```python
from build123d import *

# Parameters (mm, degrees)
F0_R          = 30
F0_R_2        = 3.625
F0_R_3        = 11.1
F2_DEPTH      = 3.25
F2_DEPTH_BACK = 3.25
F1_R          = 40
F1_R_2        = 30
F3_DEPTH      = 5
F3_DEPTH_BACK = 5


with BuildPart() as f2:
    # F0 (on Top) → F2 (new body, two sides)
    with BuildSketch(Plane.XY) as f2_sk:
        Circle(F0_R)
        with Locations((-6.983624, -20.439105)):
            Circle(F0_R_2, mode=Mode.SUBTRACT)
        with Locations((-20.439105, -6.983624)):
            Circle(F0_R_2, mode=Mode.SUBTRACT)
        with Locations((-11.348298, -11.348298)):
            Circle(F0_R_2, mode=Mode.SUBTRACT)
        with Locations((0, -24.759192)):
            Circle(F0_R_2, mode=Mode.SUBTRACT)
        with Locations((6.983624, -20.439105)):
            Circle(F0_R_2, mode=Mode.SUBTRACT)
        with Locations((0, -16.048918)):
            Circle(F0_R_2, mode=Mode.SUBTRACT)
        with Locations((11.348298, -11.348298)):
            Circle(F0_R_2, mode=Mode.SUBTRACT)
        with Locations((20.439105, -6.983624)):
            Circle(F0_R_2, mode=Mode.SUBTRACT)
        with Locations((-24.759192, 0)):
            Circle(F0_R_2, mode=Mode.SUBTRACT)
        with Locations((-16.048918, 0)):
            Circle(F0_R_2, mode=Mode.SUBTRACT)
        with Locations((-20.439105, 6.983624)):
            Circle(F0_R_2, mode=Mode.SUBTRACT)
        with Locations((-11.348298, 11.348298)):
            Circle(F0_R_2, mode=Mode.SUBTRACT)
        with Locations((-6.983624, 20.439105)):
            Circle(F0_R_2, mode=Mode.SUBTRACT)
        Circle(F0_R_3, mode=Mode.SUBTRACT)
        with Locations((11.348298, 11.348298)):
            Circle(F0_R_2, mode=Mode.SUBTRACT)
        with Locations((16.048918, 0)):
            Circle(F0_R_2, mode=Mode.SUBTRACT)
        with Locations((20.439105, 6.983624)):
            Circle(F0_R_2, mode=Mode.SUBTRACT)
        with Locations((24.759192, 0)):
            Circle(F0_R_2, mode=Mode.SUBTRACT)
        with Locations((0, 16.048918)):
            Circle(F0_R_2, mode=Mode.SUBTRACT)
        with Locations((6.983624, 20.439105)):
            Circle(F0_R_2, mode=Mode.SUBTRACT)
        with Locations((0, 24.759192)):
            Circle(F0_R_2, mode=Mode.SUBTRACT)
    extrude(amount=F2_DEPTH)
    extrude(f2_sk.sketch, amount=-F2_DEPTH_BACK)

    # F1 (on Top) → F3 (join, two sides)
    with BuildSketch(Plane.XY) as f3_sk:
        Circle(F1_R)
        Circle(F1_R_2, mode=Mode.SUBTRACT)
    extrude(amount=F3_DEPTH)
    extrude(f3_sk.sketch, amount=-F3_DEPTH_BACK)


solid = f2.part
```
For this review, take the finished solid that the model builds, in its own axes (mm). A direction names the side the tool comes from. Round coordinates to 2 decimals unless told otherwise and drop trailing zeros. Loops run counter-clockwise (first coordinate to the right, second up) from the corner with the lowest first, then second, coordinate; pieces in that order, holes last.
Q1. Insertion check: pin 1 Ø9.5 at (x, y) = (-20.44, 6.98) entering from +Z; pin 2 Ø4 at (x, z) = (-2, 1.5) entering from +Y; pin 3 Ø3 at (y, z) = (-30, -1.5) entering from -X. Each pin has a flat end and moves straight along its axis. Give the tip position at first contact, or say it passes through.
Result sheet:
pin 1: stops at z = 3.25
pin 2: stops at y = 40
pin 3: stops at x = -28.07
Q2. Add section D-D on y = -32. Write out the cut boundary in (x, z).
Result sheet:
outline: (-24, -5) - (24, -5) - (24, 5) - (-24, 5) - close
Q3. Mouldability with a two-part tool opening along Y and no side actions: class faces 3 (the face through (6, -13, 3.25)), 4 (the face through (6, 30, -5)), 5 (the face through (-8.67, -39.05, 0.07)), 6 (the face through (-29.97, 1.32, 4.11)) as +Y half, -Y half, draft (parallel to the pull), parting line (faces both ways), or undercut.
Result sheet:
face 3: undercut
face 4: draft
face 5: parting line
face 6: undercut
Q4. Machinability: for faces 1 (the face through (1.67, 21.54, -0.05)), 2 (the face through (-29.97, 1.32, -4.11)), which of the approach directions +Z, -Z, +X, -X, +Y, -Y give a long, thin tool a straight path to every point of the face, cutting with its end or side? Answer none if there is none.
Result sheet:
face 1: +Z, -Z
face 2: -Z
Q5. To check wall thickness, follow line 1 along Y through (x, z) = (13, -3); line 2 along Y through (x, z) = (-7, -1.75); line 3 along X through (y, z) = (-14.5, -2). State the ranges of each line that lie inside material, in increasing order.
Result sheet:
line 1: y = -37.83 to -14.58, -8.12 to -1.96, 1.96 to 8.12, 14.58 to 37.83
line 2: y = -39.38 to -24.06, -16.81 to -8.61, 8.61 to 16.81, 24.06 to 39.38
line 3: x = -37.28 to -13.14, -9.56 to -3.28, 3.28 to 9.56, 13.14 to 37.28
Q6. Add section A-A on y = 0. Give the number of separate pieces and of enclosed holes in the cut face, plus the area to 3 significant figures.
Result sheet:
separate pieces: 6
enclosed holes: 0
area: 257 mm2
